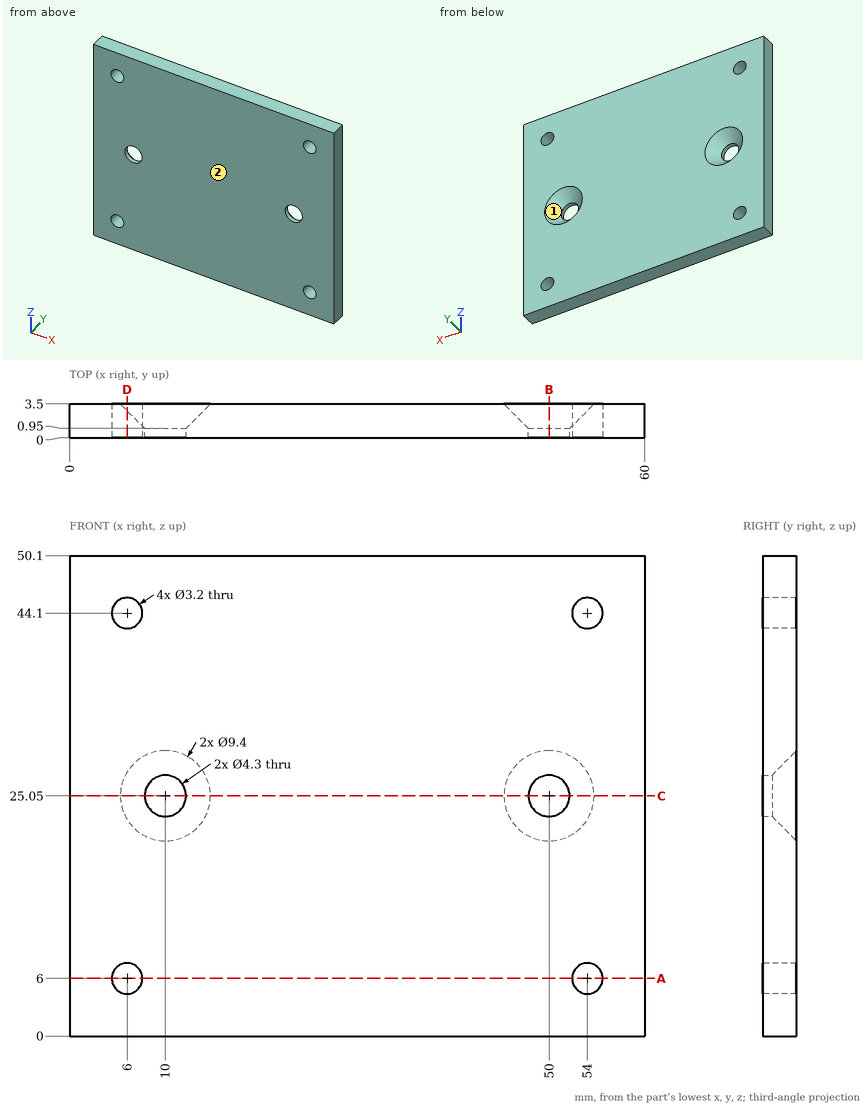
Study the drawing (mm; zero at the part's minimum x, y, z) and answer. Round coordinates to 2 decimals unless told otherwise and drop trailing zeros. Loops run counter-clockwise (first coordinate to the right, second up) from the corner with the lowest first, then second, coordinate; pieces in that order, holes last. Notation, with made-up numbers: (3, 84.25) - (24, 84.25) arc R32 ccw to (24, 119.25) - close; hole circle Ø5 at (41, 5). An arc over 180 degrees is marked (long way). Use one line per item in the form item = value. Start each with the question number.
1. For a pull along X with two mould halves and no side action, classify the marked faces 1 and 2 as pulls with the +X half, pulls with the -X half, needs draft (parallel to the pull), parting line crosses it, or undercut.
2. The part is cut by section C-C on z = 25.05. Determine the outline of the cut face in (x, y).
3. Consider line 1 (Z direction, x = 54, y = 2.55); line 2 (X direction, y = 0.4, z = 25.05); line 3 (Z direction, x = 50, y = 0.5). Determine where each line is inside the solid, lowest interval first. Write a range as [from, to].
4. The part is cut by section D-D on x = 6. Give the number of separate pieces and of enclosed holes in the cut face, then the cut area to 3 significant figures.
5. The part is cut by section B-B on x = 50. Determine the outline of the cut face in (y, z).
6. Given pin 1 Ø5 at (x, z) = (50, 25.05) entering from +Y; pin 2 Ø5.5 at (x, z) = (10, 25.05) entering from +Y, each flat-ended and moving along its own axis, determine where each tip first touches the part or whether it passes through.
7. The part is cut by section A-A on z = 6. Determine the outline of the cut face in (x, y).
Geometry check:
q1.face_1 = undercut
q1.face_2 = needs draft
q2.outline = (0, 0) - (7.85, 0) - (7.85, 0.95) - (5.3, 3.5) - (0, 3.5) - close; (12.15, 0) - (47.85, 0) - (47.85, 0.95) - (45.3, 3.5) - (14.7, 3.5) - (12.15, 0.95) - close; (52.15, 0) - (60, 0) - (60, 3.5) - (54.7, 3.5) - (52.15, 0.95) - close
q3.line_1 = [0, 4.4], [7.6, 42.5], [45.7, 50.1]
q3.line_2 = [0, 7.85], [12.15, 47.85], [52.15, 60]
q3.line_3 = [0, 22.9], [27.2, 50.1]
q4.separate_pieces = 3
q4.enclosed_holes = 0
q4.area = 151 mm^2
q5.outline = (0, 0) - (3.5, 0) - (3.5, 20.35) - (0.95, 22.9) - (0, 22.9) - close; (0, 27.2) - (0.95, 27.2) - (3.5, 29.75) - (3.5, 50.1) - (0, 50.1) - close
q6.pin_1 = 1.3
q6.pin_2 = 1.55
q7.outline = (0, 0) - (4.4, 0) - (4.4, 3.5) - (0, 3.5) - close; (7.6, 0) - (52.4, 0) - (52.4, 3.5) - (7.6, 3.5) - close; (55.6, 0) - (60, 0) - (60, 3.5) - (55.6, 3.5) - close
